The listing builds one solid part. Answer for the finished solid, in the listing's coordinates (mm). Give positions to 0.01 mm unless a question says otherwise; leave off trailing zeros. Write each loop counter-clockwise with the first axis right and the second up, starting at its lowest first coordinate (ties: lowest second). Pieces come first, ordered by that corner, then holes. Notation, with made-up numbers: (52.5, -9) - (89.5, -9) arc R23 cw to (89.5, 16) - close; hole circle Ø3 at (20.25, 34). An arc over 180 degrees is marked (long way). Answer in a Markdown table with one row per item. Add a question column.
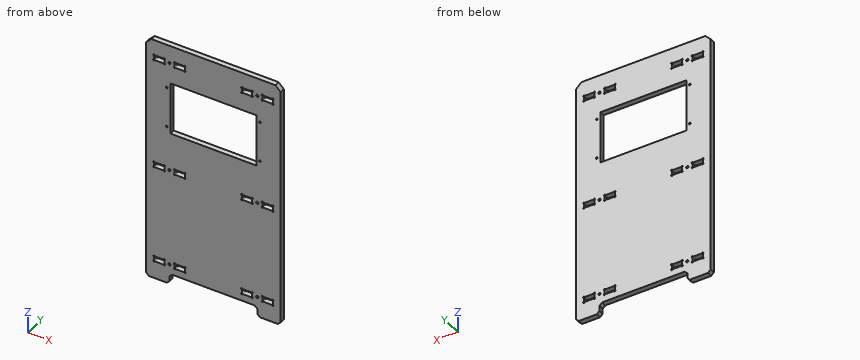
from build123d import *

# Parameters (mm, degrees)
SKETCH1_W            = 260
SKETCH1_H            = 440
EXTRUDE1_DEPTH       = 10
SKETCH3_W            = 260
SKETCH3_H            = 40
EXTRUDE3_DEPTH       = 10
SKETCH4_W            = 20
SKETCH4_H            = 10
CUT_EXTRUDE1_DEPTH   = 10
EXTRUDE4_DEPTH       = 10
MIRROR2_COPY_1_DEPTH = 10
MIRROR3_COPY_1_DEPTH = 10
MIRROR3_COPY_2_DEPTH = 10
MIRROR3_COPY_3_DEPTH = 10
MIRROR4_COPY_1_DEPTH = 10
MIRROR4_COPY_2_DEPTH = 10
MIRROR4_COPY_3_DEPTH = 10
M4_CLEARANCE_HOLE1_D = 4.5
SKETCH8_W            = 166.3
SKETCH8_H            = 101.4
CUT_EXTRUDE2_DEPTH   = 10
SKETCH9_R            = 1.75
CUT_EXTRUDE3_DEPTH   = 10
CHAMFER1_SIZE        = 10
SKETCH10_W           = 170
SKETCH10_H           = 20
EXTRUDE6_DEPTH       = 10
CHAMFER2_SIZE        = 5


with BuildPart() as part:
    # Sketch1 → Extrude1 (new body)
    with BuildSketch(Plane(origin=(0, 0, 0), x_dir=(1, 0, 0), z_dir=(0, 1, 0))):
        Rectangle(SKETCH1_W, SKETCH1_H)
    extrude(amount=EXTRUDE1_DEPTH)

    # Sketch3 → Extrude3 (add)
    with BuildSketch(Plane(origin=(0, 10, 0), x_dir=(1, 0, 0), z_dir=(0, 1, 0))):
        with Locations((0, 240)):
            Rectangle(SKETCH3_W, SKETCH3_H)
    extrude(amount=-EXTRUDE3_DEPTH)

    # Sketch4 → Cut-Extrude1 (cut)
    with BuildSketch(Plane(origin=(130, 0, -206), x_dir=(1, 0, 0), z_dir=(0, -1, 0))):
        with Locations((-235, 391)):
            Rectangle(SKETCH4_W, SKETCH4_H)
        with Locations((-195, 391)):
            Rectangle(SKETCH4_W, SKETCH4_H)
        with Locations((-65, 391)):
            Rectangle(SKETCH4_W, SKETCH4_H)
        with Locations((-25, 391)):
            Rectangle(SKETCH4_W, SKETCH4_H)
        with Locations((-235, 175)):
            Rectangle(SKETCH4_W, SKETCH4_H)
        with Locations((-195, 175)):
            Rectangle(SKETCH4_W, SKETCH4_H)
        with Locations((-65, 175)):
            Rectangle(SKETCH4_W, SKETCH4_H)
        with Locations((-25, 175)):
            Rectangle(SKETCH4_W, SKETCH4_H)
        with Locations((-235, -15)):
            Rectangle(SKETCH4_W, SKETCH4_H)
        with Locations((-195, -15)):
            Rectangle(SKETCH4_W, SKETCH4_H)
        with Locations((-65, -15)):
            Rectangle(SKETCH4_W, SKETCH4_H)
        with Locations((-25, -15)):
            Rectangle(SKETCH4_W, SKETCH4_H)
    extrude(amount=-CUT_EXTRUDE1_DEPTH, mode=Mode.SUBTRACT)

    # Sketch5 → Extrude4 (cut)
    with BuildSketch(Plane(origin=(0, 0, 0), x_dir=(-1, 0, 0), z_dir=(0, -1, 0))):
        with BuildLine():
            Line((96.5, -190), (95, -190))
            Line((95, -190), (95, -188.5))
            ThreePointArc((95, -188.5), (93.939339828, -191.060660172), (96.5, -190))
        make_face()
        with BuildLine():
            Line((115, -190), (113.5, -190))
            ThreePointArc((113.5, -190), (116.060660172, -191.060660172), (115, -188.5))
            Line((115, -188.5), (115, -190))
        make_face()
        with BuildLine():
            Line((115, -180), (113.5, -180))
            ThreePointArc((113.5, -180), (116.060660172, -178.939339828), (115, -181.5))
            Line((115, -181.5), (115, -180))
        make_face()
        with BuildLine():
            Line((96.5, -180), (95, -180))
            Line((95, -180), (95, -181.5))
            ThreePointArc((95, -181.5), (93.939339828, -178.939339828), (96.5, -180))
        make_face()
    extrude4 = extrude(amount=-EXTRUDE4_DEPTH, mode=Mode.SUBTRACT)

    # Mirror1: Extrude4 across plane
    add(extrude4.mirror(Plane(origin=(-85, 0, 0), x_dir=(0, 0, 1), z_dir=(1, 0, 0))), mode=Mode.SUBTRACT)

    # Mirror2: Extrude4 across plane
    add(extrude4.mirror(Plane(origin=(0, 0, 0), x_dir=(0, 0, 1), z_dir=(1, 0, 0))), mode=Mode.SUBTRACT)

    # Mirror2 copy 1 sketch → Mirror2 copy 1 (cut)
    with BuildSketch(Plane(origin=(170, 0, 0), x_dir=(-1, 0, 0), z_dir=(0, -1, 0))):
        with BuildLine():
            Line((96.5, -190), (95, -190))
            Line((95, -190), (95, -188.5))
            ThreePointArc((95, -188.5), (93.939339828, -191.060660172), (96.5, -190))
        make_face()
        with BuildLine():
            Line((115, -190), (113.5, -190))
            ThreePointArc((113.5, -190), (116.060660172, -191.060660172), (115, -188.5))
            Line((115, -188.5), (115, -190))
        make_face()
        with BuildLine():
            Line((115, -180), (113.5, -180))
            ThreePointArc((113.5, -180), (116.060660172, -178.939339828), (115, -181.5))
            Line((115, -181.5), (115, -180))
        make_face()
        with BuildLine():
            Line((96.5, -180), (95, -180))
            Line((95, -180), (95, -181.5))
            ThreePointArc((95, -181.5), (93.939339828, -178.939339828), (96.5, -180))
        make_face()
    extrude(amount=-MIRROR2_COPY_1_DEPTH, mode=Mode.SUBTRACT)

    # Mirror3: Extrude4 across plane
    add(extrude4.mirror(Plane(origin=(0, 0, 77), x_dir=(1, 0, 0), z_dir=(0, 0, -1))), mode=Mode.SUBTRACT)

    # Mirror3 copy 1 sketch → Mirror3 copy 1 (cut)
    with BuildSketch(Plane(origin=(-170, 0, 154), x_dir=(1, 0, 0), z_dir=(0, -1, 0))):
        with BuildLine():
            Line((96.5, -190), (95, -190))
            Line((95, -190), (95, -188.5))
            ThreePointArc((95, -188.5), (93.939339828, -191.060660172), (96.5, -190))
        make_face()
        with BuildLine():
            Line((115, -190), (113.5, -190))
            ThreePointArc((113.5, -190), (116.060660172, -191.060660172), (115, -188.5))
            Line((115, -188.5), (115, -190))
        make_face()
        with BuildLine():
            Line((115, -180), (113.5, -180))
            ThreePointArc((113.5, -180), (116.060660172, -178.939339828), (115, -181.5))
            Line((115, -181.5), (115, -180))
        make_face()
        with BuildLine():
            Line((96.5, -180), (95, -180))
            Line((95, -180), (95, -181.5))
            ThreePointArc((95, -181.5), (93.939339828, -178.939339828), (96.5, -180))
        make_face()
    extrude(amount=-MIRROR3_COPY_1_DEPTH, mode=Mode.SUBTRACT)

    # Mirror3 copy 2 sketch → Mirror3 copy 2 (cut)
    with BuildSketch(Plane(origin=(0, 0, 154), x_dir=(1, 0, 0), z_dir=(0, -1, 0))):
        with BuildLine():
            Line((96.5, -190), (95, -190))
            Line((95, -190), (95, -188.5))
            ThreePointArc((95, -188.5), (93.939339828, -191.060660172), (96.5, -190))
        make_face()
        with BuildLine():
            Line((115, -190), (113.5, -190))
            ThreePointArc((113.5, -190), (116.060660172, -191.060660172), (115, -188.5))
            Line((115, -188.5), (115, -190))
        make_face()
        with BuildLine():
            Line((115, -180), (113.5, -180))
            ThreePointArc((113.5, -180), (116.060660172, -178.939339828), (115, -181.5))
            Line((115, -181.5), (115, -180))
        make_face()
        with BuildLine():
            Line((96.5, -180), (95, -180))
            Line((95, -180), (95, -181.5))
            ThreePointArc((95, -181.5), (93.939339828, -178.939339828), (96.5, -180))
        make_face()
    extrude(amount=-MIRROR3_COPY_2_DEPTH, mode=Mode.SUBTRACT)

    # Mirror3 copy 3 sketch → Mirror3 copy 3 (cut)
    with BuildSketch(Plane(origin=(170, 0, 154), x_dir=(-1, 0, 0), z_dir=(0, -1, 0))):
        with BuildLine():
            Line((96.5, 190), (95, 190))
            Line((95, 190), (95, 188.5))
            ThreePointArc((95, 188.5), (93.939339828, 191.060660172), (96.5, 190))
        make_face()
        with BuildLine():
            Line((115, 190), (113.5, 190))
            ThreePointArc((113.5, 190), (116.060660172, 191.060660172), (115, 188.5))
            Line((115, 188.5), (115, 190))
        make_face()
        with BuildLine():
            Line((115, 180), (113.5, 180))
            ThreePointArc((113.5, 180), (116.060660172, 178.939339828), (115, 181.5))
            Line((115, 181.5), (115, 180))
        make_face()
        with BuildLine():
            Line((96.5, 180), (95, 180))
            Line((95, 180), (95, 181.5))
            ThreePointArc((95, 181.5), (93.939339828, 178.939339828), (96.5, 180))
        make_face()
    extrude(amount=-MIRROR3_COPY_3_DEPTH, mode=Mode.SUBTRACT)

    # Mirror4: Extrude4 across plane
    add(extrude4.mirror(Plane.XY.offset(-18)), mode=Mode.SUBTRACT)

    # Mirror4 copy 1 sketch → Mirror4 copy 1 (cut)
    with BuildSketch(Plane(origin=(-170, 0, -36), x_dir=(1, 0, 0), z_dir=(0, -1, 0))):
        with BuildLine():
            Line((96.5, -190), (95, -190))
            Line((95, -190), (95, -188.5))
            ThreePointArc((95, -188.5), (93.939339828, -191.060660172), (96.5, -190))
        make_face()
        with BuildLine():
            Line((115, -190), (113.5, -190))
            ThreePointArc((113.5, -190), (116.060660172, -191.060660172), (115, -188.5))
            Line((115, -188.5), (115, -190))
        make_face()
        with BuildLine():
            Line((115, -180), (113.5, -180))
            ThreePointArc((113.5, -180), (116.060660172, -178.939339828), (115, -181.5))
            Line((115, -181.5), (115, -180))
        make_face()
        with BuildLine():
            Line((96.5, -180), (95, -180))
            Line((95, -180), (95, -181.5))
            ThreePointArc((95, -181.5), (93.939339828, -178.939339828), (96.5, -180))
        make_face()
    extrude(amount=-MIRROR4_COPY_1_DEPTH, mode=Mode.SUBTRACT)

    # Mirror4 copy 2 sketch → Mirror4 copy 2 (cut)
    with BuildSketch(Plane(origin=(0, 0, -36), x_dir=(1, 0, 0), z_dir=(0, -1, 0))):
        with BuildLine():
            Line((96.5, -190), (95, -190))
            Line((95, -190), (95, -188.5))
            ThreePointArc((95, -188.5), (93.939339828, -191.060660172), (96.5, -190))
        make_face()
        with BuildLine():
            Line((115, -190), (113.5, -190))
            ThreePointArc((113.5, -190), (116.060660172, -191.060660172), (115, -188.5))
            Line((115, -188.5), (115, -190))
        make_face()
        with BuildLine():
            Line((115, -180), (113.5, -180))
            ThreePointArc((113.5, -180), (116.060660172, -178.939339828), (115, -181.5))
            Line((115, -181.5), (115, -180))
        make_face()
        with BuildLine():
            Line((96.5, -180), (95, -180))
            Line((95, -180), (95, -181.5))
            ThreePointArc((95, -181.5), (93.939339828, -178.939339828), (96.5, -180))
        make_face()
    extrude(amount=-MIRROR4_COPY_2_DEPTH, mode=Mode.SUBTRACT)

    # Mirror4 copy 3 sketch → Mirror4 copy 3 (cut)
    with BuildSketch(Plane(origin=(170, 0, -36), x_dir=(-1, 0, 0), z_dir=(0, -1, 0))):
        with BuildLine():
            Line((96.5, 190), (95, 190))
            Line((95, 190), (95, 188.5))
            ThreePointArc((95, 188.5), (93.939339828, 191.060660172), (96.5, 190))
        make_face()
        with BuildLine():
            Line((115, 190), (113.5, 190))
            ThreePointArc((113.5, 190), (116.060660172, 191.060660172), (115, 188.5))
            Line((115, 188.5), (115, 190))
        make_face()
        with BuildLine():
            Line((115, 180), (113.5, 180))
            ThreePointArc((113.5, 180), (116.060660172, 178.939339828), (115, 181.5))
            Line((115, 181.5), (115, 180))
        make_face()
        with BuildLine():
            Line((96.5, 180), (95, 180))
            Line((95, 180), (95, 181.5))
            ThreePointArc((95, 181.5), (93.939339828, 178.939339828), (96.5, 180))
        make_face()
    extrude(amount=-MIRROR4_COPY_3_DEPTH, mode=Mode.SUBTRACT)

    # M4 Clearance Hole1 (through all)
    with Locations(Plane(origin=(0, 10, 0), x_dir=(1, 0, 0), z_dir=(0, 1, 0))):
        with Locations((-85, 221), (85, 221), (85, 31), (-85, 31), (-85, -185), (85, -185)):
            Hole(M4_CLEARANCE_HOLE1_D / 2)

    # Sketch8 → Cut-Extrude2 (cut)
    with BuildSketch(Plane(origin=(130, 0, -206), x_dir=(1, 0, 0), z_dir=(0, -1, 0))):
        with Locations((-130, 300.3)):
            Rectangle(SKETCH8_W, SKETCH8_H)
    extrude(amount=-CUT_EXTRUDE2_DEPTH, mode=Mode.SUBTRACT)

    # Sketch9 → Cut-Extrude3 (cut)
    with BuildSketch(Plane(origin=(-103.5, 10, 155.65), x_dir=(-1, 0, 0), z_dir=(0, 1, 0))):
        with Locations(Location((-13.45, -22.05, 0), (0, 0, 90))):
            Circle(SKETCH9_R)
        with Locations(Location((-193.55, -22.05, 0), (0, 0, 90))):
            Circle(SKETCH9_R)
        with Locations(Location((-13.45, -100.65, 0), (0, 0, 90))):
            Circle(SKETCH9_R)
        with Locations(Location((-193.55, -100.55, 0), (0, 0, 90))):
            Circle(SKETCH9_R)
    extrude(amount=-CUT_EXTRUDE3_DEPTH, mode=Mode.SUBTRACT)

    # Chamfer1
    chamfer1_edges = [part.edges().sort_by_distance(p)[0] for p in [
        (130, 5, 220),
        (-130, 5, 220),
    ]]
    chamfer(chamfer1_edges, length=CHAMFER1_SIZE)

    # Sketch10 → Extrude6 (cut)
    with BuildSketch(Plane.XZ):
        with Locations((0, -250)):
            Rectangle(SKETCH10_W, SKETCH10_H)
    extrude(amount=-EXTRUDE6_DEPTH, mode=Mode.SUBTRACT)

    # Chamfer2
    chamfer2_edges = [part.edges().sort_by_distance(p)[0] for p in [
        (-130, 5, -260),
        (130, 5, -260),
        (-85, 5, -260),
        (-85, 5, -240),
        (85, 5, -240),
        (85, 5, -260),
    ]]
    chamfer(chamfer2_edges, length=CHAMFER2_SIZE)


solid = part.part
1. Straight lines are drawn through the part: L1, parallel to Z at x = -63, y = 7.5; L2, parallel to Z at x = -55.5, y = 5; L3, parallel to Z at x = -102.5, y = 3.5. For each, find the intervals that lie inside material, in ascending order. Write a range as [from, to].
2. Section A-A (x = 14) is taken. Give the vertices of the cut face in (y, z), and give its area (3 significant figures).
3. Given pin 1 Ø4 at (x, z) = (59, -164.5) entering from -Y; pin 2 Ø2.5 at (x, z) = (95, -226) entering from -Y; pin 3 Ø1 at (x, y) = (29.5, 7) entering from -Z, each flat-ended and moving along its own axis, determine where each tip first touches the part or whether it passes through.
4. Section B-B (y = 3.25) is taken. State how many separate pieces and enclosed holes the cut face has, and give its area (3 significant figures).
Geometry check:
| question | item | result |
|---|---|---|
| 1 | L1 | [-240, -226], [-216, -36], [-26, 43.6], [145, 180], [190, 220] |
| 1 | L2 | [-240, -227.41], [-214.59, -37.41], [-24.59, 43.6], [145, 178.59], [191.41, 220] |
| 1 | L3 | [-260, -226], [-216, -36], [-26, 180], [190, 220] |
| 2 | outline | (0, -240) - (10, -240) - (10, 43.6) - (0, 43.6) - close; (0, 145) - (10, 145) - (10, 220) - (0, 220) - close |
| 2 | area | 3,590 mm² |
| 3 | pin 1 | y = 0 |
| 3 | pin 2 | through |
| 3 | pin 3 | z = -240 |
| 4 | separate pieces | 1 |
| 4 | enclosed holes | 23 |
| 4 | area | 102,000 mm² |
